Autodesk Fusion 360 part; units mm, degrees
sketch "Sketch1" plane through (0, 0, 0) normal (0, 1, 0) x (1, 0, 0)
  line L0 (0, 0) -> (0, 150)
  line L1 (260, 410) -> (410, 410)
  arc A0 (260, 410) -> (0, 150) centre (260, 150) ccw
  point P0 (0, 410)
  dimension "d1" = 410
  dimension "d2" = 410
  dimension "d3" = 260
sketch "Sketch2" plane through (0, 0, 0) normal (0, 0, 1) x (1, 0, 0)
  circle A0 centre (0, 0) radius 145
  circle A1 centre (0, 0) radius 105
  dimension "d4" = 290
  dimension "d5" = 210
sweep "Sweep1" add profiles "Sketch2" path "Sketch1" along L1 A0 L0 section 1
sketch "Sketch3" plane through (0, 0, 0) normal (0, 0, 1) x (-1, 0, 0)
  circle A0 centre (0, 0) radius 105
  circle A1 centre (0, 0) radius 145
  line L0 (-180, 180) -> (180, 180)
  line L1 (180, 180) -> (180, -180)
  line L2 (180, -180) -> (-180, -180)
  line L3 (-180, -180) -> (-180, 180)
  line L4 (-180, 180) -> (180, -180) construction
  line L5 (180, 180) -> (-180, -180) construction
  dimension "d12" = 360
  dimension "d13" = 360
extrude "Extrude1" add sketch "Sketch3" against normal blind 50 contours L0 L1 L2 L3
sketch "Sketch4" plane through (410, 0, 0) normal (1, 0, 0) x (0, 1, 0)
  circle A0 centre (0, -410) radius 105
  circle A1 centre (0, -410) radius 145
  line L0 (180, -580) -> (-180, -580)
  line L1 (-180, -580) -> (-180, -220)
  line L2 (-180, -220) -> (180, -220)
  line L3 (180, -220) -> (180, -580)
  line L4 (180, -580) -> (-180, -220) construction
  line L5 (-180, -580) -> (180, -220) construction
  point P0 (0, -400)
  dimension "d16" = 360
  dimension "d17" = 360
extrude "Extrude2" add sketch "Sketch4" against normal blind 50 contours L0 L1 L2 L3
fillet "Fillet1" radius 20 4 edges at (180, -180, -25) (180, 180, -25) (-180, -180, -25) (-180, 180, -25)
fillet "Fillet2" radius 20 4 edges at (385, -180, -220) (385, 180, -220) (385, 180, -580) (385, -180, -580)
fillet "Fillet3" radius 10 2 edges at (-135.1875, 52.4342, -50) (360, -52.4342, -545.1875)
sketch "Sketch5" plane through (0, 0, 0) normal (0, 0, 1) x (-1, 0, 0)
  arc A0 (160, -180) -> (180, -160) centre (160, -160) ccw
  line L0 (180, -160) -> (180, 160)
  arc A1 (180, 160) -> (160, 180) centre (160, 160) ccw
  line L1 (160, 180) -> (-160, 180)
  arc A2 (-160, 180) -> (-180, 160) centre (-160, 160) ccw
  line L2 (-180, 160) -> (-180, -160)
  arc A3 (-180, -160) -> (-160, -180) centre (-160, -160) ccw
  line L3 (-160, -180) -> (160, -180)
  circle A4 centre (0, 0) radius 105
  line L4 (130, 130) -> (-130, 130) construction
  line L5 (-130, 130) -> (-130, -130) construction
  line L6 (-130, -130) -> (130, -130) construction
  line L7 (130, -130) -> (130, 130) construction
  line L8 (130, 130) -> (-130, -130) construction
  line L9 (-130, 130) -> (130, -130) construction
  dimension "d26" = 260
  dimension "d27" = 260
hole "Hole1" at (130, 130, 0) at (-130, 130, 0) at (-130, -130, 0) at (130, -130, 0) direction (0, 0, -1) diameter 30 depth 50 tip angle 180 counterbore diameter 60 counterbore depth 10
sketch "Sketch6" plane through (410, 0, 0) normal (1, 0, 0) x (0, 1, 0)
  arc A0 (-180, -560) -> (-160, -580) centre (-160, -560) ccw
  line L0 (-160, -580) -> (160, -580)
  arc A1 (160, -580) -> (180, -560) centre (160, -560) ccw
  line L1 (180, -560) -> (180, -240)
  arc A2 (180, -240) -> (160, -220) centre (160, -240) ccw
  line L2 (160, -220) -> (-160, -220)
  arc A3 (-160, -220) -> (-180, -240) centre (-160, -240) ccw
  line L3 (-180, -240) -> (-180, -560)
  circle A4 centre (0, -410) radius 105
sketch "Sketch7" plane through (410, 0, 0) normal (1, 0, 0) x (0, 1, 0)
  line L0 (130, -270) -> (-130, -270) construction
  line L1 (-130, -270) -> (-130, -530) construction
  line L2 (-130, -530) -> (130, -530) construction
  line L3 (130, -530) -> (130, -270) construction
  line L4 (130, -270) -> (-130, -530) construction
  line L5 (-130, -270) -> (130, -530) construction
  point P0 (0, -400)
  dimension "d33" = 260
  dimension "d34" = 260
hole "Hole2" at (410, 130, -270) at (410, -130, -270) at (410, -130, -530) at (410, 130, -530) direction (-1, 0, 0) diameter 30 depth 50 tip angle 180 counterbore diameter 60 counterbore depth 10
chamfer "Chamfer1" distance 10 angle 45 2 edges at (410, -37.9696, -507.8944) (-97.8944, 37.9696, 0)
sketch "Sketch8" plane through (0, 0, 0) normal (0, 0, 1) x (-1, 0, 0)
  circle A0 centre (130, 130) radius 30
  circle A1 centre (-130, -130) radius 30
  circle A2 centre (130, -130) radius 30
  circle A3 centre (-130, 130) radius 30
  arc A4 (160, -180) -> (180, -160) centre (160, -160) ccw
  line L0 (180, -160) -> (180, 160)
  arc A5 (180, 160) -> (160, 180) centre (160, 160) ccw
  line L1 (160, 180) -> (-160, 180)
  arc A6 (-160, 180) -> (-180, 160) centre (-160, 160) ccw
  line L2 (-180, 160) -> (-180, -160)
  arc A7 (-180, -160) -> (-160, -180) centre (-160, -160) ccw
  line L3 (-160, -180) -> (160, -180)
  circle A8 centre (0, 0) radius 115
sketch "Sketch9" plane through (410, 0, 0) normal (1, 0, 0) x (0, 1, 0)
sketch "Sketch10" plane through (0, 0, 0) normal (0, 0, 1) x (-1, 0, 0)
Input: part model. Units: mm. Frame: model coordinates. A direction names the side the tool comes from. Coordinates: 2 decimals unless noted, no trailing zeros. Loops run counter-clockwise (first coordinate to the right, second up) from the corner with the lowest first, then second, coordinate; pieces in that order, holes last. Notation, with made-up numbers: (48, -28.75) -> (77, -28.75) arc R22 cw to (77, -13.75) -> close; hole circle Ø1 at (11.25, 15.5). An arc over 180 degrees is marked (long way). Write item = value, one per line. Start each with the question number.
Item 1: Material intervals for line 1 (Y direction, x = 404, z = -270); line 2 (Y direction, x = 130, z = -31); line 3 (Z direction, x = 387, y = -130), sorted ascending.
Item 2: Cut plane C-C, the plane y = -130. Count the separate pieces of the cut face and the enclosed holes in it, plus the area to 3 significant figures.
Item 3: Cut plane B-B, the plane x = 323. Return loops of the section in (y, z).
Item 4: Reachability of faces 1 (the face through (400, 136, -256)), 2 (the face through (385, -2, -220)), 3 (the face through (360, -83, -277)) from +Z, -Z, +X, -X, +Y, -Y: full face, straight path, thin tool, end or side. Return the list, or none.
Item 5: First-contact query: P1, Ø18, axis at y = 130, z = -535, coming from the +X side; P2, Ø18, axis at x = -124.5, y = -122, coming from the +Z side; P3, Ø5, axis at x = 293, y = -124.5, coming from the +Z side; P4, Ø2, axis at x = 309.5, z = -479, coming from the +Y side. Flat tips, straight axial feed; report the tip coordinate or a pass-through.
Item 6: Mould query, pull axis Y, two halves, no side actions, for faces 4 (the face through (173.986, 174.297, -25.35)), 5 (the face through (305.63, -43.554, -271.696)), 6 (the face through (-100.713, 136.503, -5.07)), 7 (the face through (-144, -136, -10)). Classes: pulls with the +Y half, pulls with the -Y half, needs draft (parallel to the pull), parting line crosses it, or undercut.
Ans:
q1.line_1 = -180 to -160, -100 to 100, 160 to 180
q1.line_2 = -180 to -145, -115 to 115, 145 to 180
q1.line_3 = -580 to -545, -515 to -285, -255 to -220
q2.separate_pieces = 5
q2.enclosed_holes = 0
q2.area = 107,000 mm²
q3.outline = circle Ø290 at (0, -410); hole circle Ø210 at (0, -410)
q4.face_1 = +X
q4.face_2 = +Z, +X, +Y, -Y
q4.face_3 = none
q5.P1 = through
q5.P2 = -10
q5.P3 = -331.64
q5.P4 = 128.07
q6.face_4 = pulls with the +Y half
q6.face_5 = parting line crosses it
q6.face_6 = undercut
q6.face_7 = undercut
